Work out the finished part from the listing and answer in its coordinate system (mm). A direction names the side the tool comes from. Coordinates: 2 decimals unless noted, no trailing zeros. Order: outer loops, then holes, each group sorted by start corner. A loop starts at its lowest first (then second) coordinate and runs counter-clockwise, first axis right, second up. Notation, with made-up numbers: M -0.75,28 L 24.25,28 A30 ccw 24.25,63 Z; hole C 5.25,3.25 d9. An arc over 180 degrees is marked long. Use a Markdown table: item, result. Add a question column.
from build123d import *

# Parameters (mm, degrees)
EXTRUDE_6_DEPTH      = 39
CUT_EXTRUDE_START    = 3
CUT_EXTRUDE_2_DEPTH  = 33
EXTRUDE_START        = 9.5
SKETCH_7_W           = 35
SKETCH_7_H           = 13
EXTRUDE_7_DEPTH      = 20
EXTRUDE_START_2      = -16.5
EXTRUDE_8_DEPTH      = 4
CUT_EXTRUDE_START_2  = 180
CUT_EXTRUDE_3_DEPTH  = 10
SKETCH_13_R          = 1.5
CUT_EXTRUDE_4_DEPTH  = 30
SKETCH_14_W          = 15
SKETCH_14_H          = 2
CUT_EXTRUDE_5_DEPTH  = 30
CUT_EXTRUDE_START_3  = 17
CUT_EXTRUDE_7_DEPTH  = 85
CUT_EXTRUDE_START_4  = 13
CUT_EXTRUDE_9_DEPTH  = 5
SKETCH_20_W          = 16.6
SKETCH_20_H          = 24.7
CUT_EXTRUDE_10_DEPTH = 5
SKETCH_21_R          = 6.5
CUT_EXTRUDE_11_DEPTH = 5
CUT_EXTRUDE_12_DEPTH = 17
CUT_EXTRUDE_13_DEPTH = 3
CUT_EXTRUDE_START_5  = 30
CUT_EXTRUDE_14_DEPTH = 3
SKETCH_26_W          = 12.700381469
SKETCH_26_H          = 20
EXTRUDE_9_DEPTH      = 2
EXTRUDE_START_3      = 7
SKETCH_27_W          = 17
SKETCH_27_H          = 33
EXTRUDE_10_DEPTH     = 3


with BuildPart() as part:
    # Эскиз1 → Бобышка-Вытянуть6 (new body)
    with BuildSketch(Plane.XY):
        with BuildLine():
            Line((4.299618531, 175.402841826), (4.299618531, 188.402841826))
            Line((4.299618531, 188.402841826), (75.299618531, 188.402841826))
            Line((75.299618531, 188.402841826), (96.299618531, 168.402841826))
            Line((96.299618531, 168.402841826), (96.299619, 0))
            Line((96.299619, 0), (96.299619, -28))
            Line((96.299619, -28), (0, -28))
            Line((0, -28), (0, 0))
            ThreePointArc((0, 0), (37.229295141, 21.561020186), (55.173142182, 60.662380285))
            ThreePointArc((55.173142182, 60.662380285), (56.797307883, 87.162380285), (55.173142182, 113.662380285))
            ThreePointArc((55.173142182, 113.662380285), (38.726552267, 151.940422917), (4.299618531, 175.402841826))
        make_face()
    extrude(amount=EXTRUDE_6_DEPTH)

    # Эскиз5 → Вырез-Вытянуть2 (cut)
    with BuildSketch(Plane.XY.offset(CUT_EXTRUDE_START)):
        Polygon((34.099618531, 175.402841826), (4.299618531, 175.402841826), (4.299618531, 169.021888999), (-18.700381469, 169.021888999), (-18.700381469, -25), (14, -25), (14, 6.5), (30.299619, 6.5), (30.299619, -25), (91.299619, -25), (91.299619, 169.021888999), (74.099618531, 185.402841826), (34.099618531, 185.402841826), align=None)
    extrude(amount=CUT_EXTRUDE_2_DEPTH, mode=Mode.SUBTRACT)

    # Эскиз7 → Бобышка-Вытянуть7 (add)
    with BuildSketch(Plane.XY.offset(EXTRUDE_START)):
        with Locations((-13.200381469, 181.902841826)):
            Rectangle(SKETCH_7_W, SKETCH_7_H)
    extrude(amount=EXTRUDE_7_DEPTH)

    # Эскиз22 → Бобышка-Вытянуть8 (add)
    with BuildSketch(Plane(origin=(0, 188.402841826, 0), x_dir=(1, 0, 0), z_dir=(0, 1, 0)).offset(EXTRUDE_START_2)):
        Polygon((10.299618531, -29.5), (10.299618531, -33.5375), (-12.700381469, -39), (-12.700381469, -29.5), align=None)
        Polygon((-12.700381469, -9.5), (-12.700381469, 0), (10.299618531, -5.4625), (10.299618531, -9.5), align=None)
    extrude(amount=EXTRUDE_8_DEPTH)

    # Эскиз12 → Вырез-Вытянуть3 (cut)
    with BuildSketch(Plane(origin=(0, 0, 0), x_dir=(1, 0, 0), z_dir=(0, 1, 0)).offset(CUT_EXTRUDE_START_2)):
        with BuildLine():
            Line((-7.700381469, -34.154700538), (-7.200381469, -33.866025404))
            ThreePointArc((-7.200381469, -33.866025404), (-7.700381469, -32), (-8.200381469, -33.866025404))
            Line((-8.200381469, -33.866025404), (-7.700381469, -34.154700538))
        make_face()
        with BuildLine():
            Line((-7.700381469, -7.154700538), (-7.200381469, -6.866025404))
            ThreePointArc((-7.200381469, -6.866025404), (-7.700381469, -5), (-8.200381469, -6.866025404))
            Line((-8.200381469, -6.866025404), (-7.700381469, -7.154700538))
        make_face()
    extrude(amount=-CUT_EXTRUDE_3_DEPTH, mode=Mode.SUBTRACT)

    # Эскиз13 → Вырез-Вытянуть4 (cut)
    with BuildSketch(Plane.XY):
        with Locations((-2.700381469, 183.402841826)):
            Circle(SKETCH_13_R)
    extrude(amount=CUT_EXTRUDE_4_DEPTH, mode=Mode.SUBTRACT)

    # Эскиз14 → Вырез-Вытянуть5 (cut)
    with BuildSketch(Plane.XY):
        with Locations((-23.200381469, 187.402841826)):
            Rectangle(SKETCH_14_W, SKETCH_14_H)
    extrude(amount=CUT_EXTRUDE_5_DEPTH, mode=Mode.SUBTRACT)

    # Эскиз17 → Вырез-Вытянуть7 (cut)
    with BuildSketch(Plane(origin=(0, 0, 0), x_dir=(0, 0, -1), z_dir=(1, 0, 0)).offset(CUT_EXTRUDE_START_3)):
        with BuildLine():
            Line((-24.118802154, -2.5), (-22.964101615, -0.5))
            ThreePointArc((-22.964101615, -0.5), (-15.5, -2.5), (-22.964101615, -4.5))
            Line((-22.964101615, -4.5), (-24.118802154, -2.5))
        make_face()
    extrude(amount=CUT_EXTRUDE_7_DEPTH, mode=Mode.SUBTRACT)

    # Эскиз18 → Вырез-Вытянуть9 (cut)
    with BuildSketch(Plane(origin=(0, 0, 0), x_dir=(0, 0, -1), z_dir=(1, 0, 0)).offset(CUT_EXTRUDE_START_4)):
        with BuildLine():
            Line((-21.809401077, -2.5), (-21.232050808, -1.5))
            ThreePointArc((-21.232050808, -1.5), (-17.5, -2.5), (-21.232050808, -3.5))
            Line((-21.232050808, -3.5), (-21.809401077, -2.5))
        make_face()
    extrude(amount=CUT_EXTRUDE_9_DEPTH, mode=Mode.SUBTRACT)

    # Эскиз20 → Вырез-Вытянуть10 (cut)
    with BuildSketch(Plane(origin=(0, 188.402841826, 0), x_dir=(1, 0, 0), z_dir=(0, 1, 0))):
        with Locations((50.95, -19.5)):
            Rectangle(SKETCH_20_W, SKETCH_20_H)
        with BuildLine():
            Line((40, -32.143375673), (40.625, -31.782531755))
            ThreePointArc((40.625, -31.782531755), (40, -29.45), (39.375, -31.782531755))
            Line((39.375, -31.782531755), (40, -32.143375673))
        make_face()
        with BuildLine():
            Line((40, -9.743375673), (40.625, -9.382531755))
            ThreePointArc((40.625, -9.382531755), (40, -7.05), (39.375, -9.382531755))
            Line((39.375, -9.382531755), (40, -9.743375673))
        make_face()
        with BuildLine():
            Line((61.9, -9.743375673), (62.525, -9.382531755))
            ThreePointArc((62.525, -9.382531755), (61.9, -7.05), (61.275, -9.382531755))
            Line((61.275, -9.382531755), (61.9, -9.743375673))
        make_face()
        with BuildLine():
            Line((61.9, -32.143375673), (62.525, -31.782531755))
            ThreePointArc((62.525, -31.782531755), (61.9, -29.45), (61.275, -31.782531755))
            Line((61.275, -31.782531755), (61.9, -32.143375673))
        make_face()
    extrude(amount=-CUT_EXTRUDE_10_DEPTH, mode=Mode.SUBTRACT)

    # Эскиз21 → Вырез-Вытянуть11 (cut)
    with BuildSketch(Plane(origin=(129.903734815, 136.398921556, 0), x_dir=(0, 0, -1), z_dir=(0.689655172, 0.724137931, 0))):
        with Locations((-19.5, 60.905684392)):
            Circle(SKETCH_21_R)
    extrude(amount=-CUT_EXTRUDE_11_DEPTH, mode=Mode.SUBTRACT)

    # Эскиз23 → Вырез-Вытянуть12 (cut)
    with BuildSketch(Plane.ZY.offset(-14)):
        with BuildLine():
            Line((22.964101615, -17), (22.098076211, -15.5))
            ThreePointArc((22.098076211, -15.5), (16.5, -17), (22.098076211, -18.5))
            Line((22.098076211, -18.5), (22.964101615, -17))
        make_face()
    extrude(amount=-CUT_EXTRUDE_12_DEPTH, mode=Mode.SUBTRACT)

    # Эскиз24 → Вырез-Вытянуть13 (cut)
    with BuildSketch(Plane.XY.offset(3)):
        Polygon((11, -1), (27.169940805, 6.907781886), (23.655371078, 14.094422244), (7.485430273, 6.186640358), align=None)
    extrude(amount=CUT_EXTRUDE_13_DEPTH, mode=Mode.SUBTRACT)

    # Эскиз25 → Вырез-Вытянуть14 (cut)
    with BuildSketch(Plane.XY.offset(3).offset(CUT_EXTRUDE_START_5)):
        Polygon((11, -1), (27.169940805, 6.907781886), (23.655371078, 14.094422244), (7.485430273, 6.186640358), align=None)
    extrude(amount=CUT_EXTRUDE_14_DEPTH, mode=Mode.SUBTRACT)

    # Эскиз26 → Бобышка-Вытянуть9 (add)
    with BuildSketch(Plane.XZ.offset(-175.402841826)):
        with Locations((-6.350190735, 19.5)):
            Rectangle(SKETCH_26_W, SKETCH_26_H)
    extrude(amount=EXTRUDE_9_DEPTH)

    # Эскиз27 → Бобышка-Вытянуть10 (add)
    with BuildSketch(Plane(origin=(127.834769298, 134.226507763, 0), x_dir=(0.724137931, -0.689655172, 0), z_dir=(-0.689655172, -0.724137931, 0)).offset(EXTRUDE_START_3)):
        with Locations((-58.953302792, 19.5)):
            Rectangle(SKETCH_27_W, SKETCH_27_H)
    extrude(amount=EXTRUDE_10_DEPTH)


solid = part.part
(1) Which of the six approach directions +Z, -Z, +X, -X, +Y, -Y give full straight-line access (tool end or side, diameter ignored) to faces 1 (the flat face through (24, 6.5, 19)), 2 (the cylindrical face through (36.816, 21.11, 1.479)), 3 (the flat face through (-23, 186.403, 19)), 4 (the flat face through (65, 82, 36)), 5 (the flat face through (-22, 175.403, 19))?
(2) A cutting plane is placed at D-D on y = 11.5. Write down the section's boundary in (x, z), plus the area to 3 significant figures.
(3) A cutting plane is placed at A-A on x = 23. Write down the section's boundary in (y, z).
(4) A cutting plane is placed at B-B on y = -10.5. Write down the section's boundary in (x, z), plus the area to 3 significant figures.
(5) A cutting plane is placed at C-C on x = 52.5. Write down the section's boundary in (y, z).
(6) Straight lines are drawn through the part: line 1 (Z direction, x = 61.9, y = 187.6); line 2 (Z direction, x = 73, y = 48); line 3 (Y direction, x = 6.5, z = 4.5). For each, find the intervals that lie inside material, in ascending order.
(7) Given P1, Ø5, axis at y = -2.5, z = 19.5, coming from the +X side; P2, Ø4, axis at x = -8.5, z = 34, coming from the +Y side; P3, Ø1.8, axis at x = -1, y = 174.5, coming from the +Z side, each flat-ended and moving along its own axis, determine where each tip first touches the part or whether it passes through.
(8) The mould has two halves that part along Z. Classify faces 6 (the flat face through (60, 82, 39)), 7 (the flat face through (7, -25, 19)), 8 (the flat face through (-4, 171.903, 33)), 9 (the flat face through (17, 175.403, 19)): pulls with the +Z half, pulls with the -Z half, needs draft (parallel to the pull), parting line crosses it, or undercut.
From the geometry:
| question | item | result |
|---|---|---|
| 1 | face 1 | -X |
| 1 | face 2 | +Z, -Z, -X |
| 1 | face 3 | +Z, -Z, -X, +Y |
| 1 | face 4 | none |
| 1 | face 5 | +Z, -Z, -X, -Y |
| 2 | outline | M 25.89,0 L 96.3,0 L 96.3,39 L 25.89,39 L 25.89,36 L 91.3,36 L 91.3,3 L 25.89,3 Z |
| 2 | area | 587 mm2 |
| 3 | outline | M -28,0 L 9.55,0 L 9.55,3 L 4.87,3 L 4.87,6 L 6.5,6 L 6.5,33 L 4.87,33 L 4.87,36 L 9.55,36 L 9.55,39 L -28,39 Z; M 166.25,0 L 188.4,0 L 188.4,39 L 166.25,39 L 166.25,36 L 175.4,36 L 175.4,3 L 166.25,3 Z; hole M -18.5,22.1 A3 ccw long -15.5,22.1 L -17,22.96 Z; hole M -4.5,22.96 A4 ccw long -0.5,22.96 L -2.5,24.12 Z |
| 4 | outline | M 0,0 L 96.3,0 L 96.3,39 L 0,39 L 0,36 L 14,36 L 14,3 L 0,3 Z; hole M 30.3,3 L 91.3,3 L 91.3,36 L 30.3,36 Z |
| 4 | area | 1,280 mm2 |
| 5 | outline | M -28,0 L 48.24,0 L 48.24,3 L -25,3 L -25,36 L 48.24,36 L 48.24,39 L -28,39 Z; M 126.27,0 L 188.4,0 L 188.4,7.15 L 185.4,7.15 L 185.4,3 L 126.27,3 Z; M 126.27,36 L 185.4,36 L 185.4,31.85 L 188.4,31.85 L 188.4,39 L 126.27,39 Z |
| 6 | line 1 | z = 0 to 7.05, 9.74 to 29.45, 32.14 to 39 |
| 6 | line 2 | z = 0 to 3, 36 to 39 |
| 6 | line 3 | y = -28 to -25, 175.4 to 188.4 |
| 7 | P1 | stops at x = 17 |
| 7 | P2 | stops at y = 175.9 |
| 7 | P3 | stops at z = 36.43 |
| 8 | face 6 | pulls with the +Z half |
| 8 | face 7 | undercut |
| 8 | face 8 | needs draft |
| 8 | face 9 | undercut |
